Work out the finished part from the listing and answer in its coordinate system (mm). A direction names the side the tool comes from. Coordinates: 2 decimals unless noted, no trailing zeros. Order: outer loops, then holes, each group sorted by start corner. A loop starts at its lowest first (then second) coordinate and runs counter-clockwise, first axis right, second up. Notation, with made-up numbers: M -10.5,22 L 4.5,22 A27 ccw 4.5,38 Z; hole C 70.5,0 d2. An arc over 180 degrees is marked long. Use a Markdown table: item, result.
from build123d import *

# Parameters (mm, degrees)
BOSS_EXTRUDE1_DEPTH     = 6.35
CUT_EXTRUDE1_DEPTH      = 244.131209432
CUT_EXTRUDE1_DEPTH_BACK = 244.131209432
SKETCH4_W               = 101.6
SKETCH4_H               = 101.6
SKETCH4_W_2             = 22.606
SKETCH4_H_2             = 3.302
SKETCH5_W               = 6.888524177
SKETCH5_H               = 88.9
CUT_EXTRUDE2_DEPTH      = 6.35
SKETCH6_R               = 1.429315601
CUT_EXTRUDE3_DEPTH      = 13.97


with BuildPart() as part:
    # Sketch3 → Boss-Extrude1 (new body)
    with BuildSketch(Plane.XY):
        Polygon((0, 77.53985), (0, 55.81015), (5.9944, 55.81015), (5.9944, 34.08045), (0, 34.08045), (0, 12.35075), (0, 0), (25.54605, 0), (25.54605, 5.9944), (47.27575, 5.9944), (47.27575, 0), (69.00545, 0), (69.00545, 5.9944), (90.73515, 5.9944), (90.73515, 0), (112.46485, 0), (112.46485, 5.9944), (134.19455, 5.9944), (134.19455, 0), (155.92425, 0), (155.92425, 5.9944), (177.65395, 5.9944), (177.65395, 0), (203.2, 0), (203.2, 34.08045), (197.2056, 34.08045), (197.2056, 55.81015), (203.2, 55.81015), (203.2, 77.53985), (197.2056, 77.53985), (197.2056, 99.26955), (203.2, 99.26955), (203.2, 120.99925), (203.2, 133.35), (177.65395, 133.35), (177.65395, 127.3556), (155.92425, 127.3556), (155.92425, 133.35), (134.19455, 133.35), (134.19455, 127.3556), (112.46485, 127.3556), (112.46485, 133.35), (90.73515, 133.35), (90.73515, 127.3556), (69.00545, 127.3556), (69.00545, 133.35), (47.27575, 133.35), (47.27575, 127.3556), (25.54605, 127.3556), (25.54605, 133.35), (0, 133.35), (0, 99.26955), (5.9944, 99.26955), (5.9944, 77.53985), align=None)
    extrude(amount=BOSS_EXTRUDE1_DEPTH)

    # Sketch4 → Cut-Extrude1 (cut, two sides: drawn at the far end of the back side and taken through both)
    with BuildSketch(Plane.XY.offset(6.35).offset(-CUT_EXTRUDE1_DEPTH_BACK)):
        with Locations((69.942028986, 69.85)):
            Rectangle(SKETCH4_W, SKETCH4_H)
        with BuildLine():
            ThreePointArc((189.068028986, 120.65), (186.020028986, 123.698), (182.972028986, 120.65))
            Line((182.972028986, 120.65), (189.068028986, 120.65))
        make_face()
        with BuildLine():
            Line((189.068028986, 120.65), (182.972028986, 120.65))
            ThreePointArc((182.972028986, 120.65), (186.020028986, 117.602), (189.068028986, 120.65))
        make_face()
        with BuildLine():
            ThreePointArc((176.368028986, 120.65), (173.320028986, 123.698), (170.272028986, 120.65))
            Line((170.272028986, 120.65), (176.368028986, 120.65))
        make_face()
        with BuildLine():
            Line((176.368028986, 120.65), (170.272028986, 120.65))
            ThreePointArc((170.272028986, 120.65), (173.320028986, 117.602), (176.368028986, 120.65))
        make_face()
        with Locations((164.557028986, 20.701)):
            Rectangle(SKETCH4_W_2, SKETCH4_H_2)
    extrude(amount=CUT_EXTRUDE1_DEPTH + CUT_EXTRUDE1_DEPTH_BACK, mode=Mode.SUBTRACT)

    # Sketch5 → Cut-Extrude2 (cut)
    with BuildSketch(Plane(origin=(0, 0, 0), x_dir=(-1, 0, 0), z_dir=(0, 0, -1))):
        with Locations((-145.073671488, 66.675)):
            Rectangle(SKETCH5_W, SKETCH5_H)
    extrude(amount=-CUT_EXTRUDE2_DEPTH, mode=Mode.SUBTRACT)

    # Sketch6 → Cut-Extrude3 (cut)
    with BuildSketch(Plane.XY.offset(6.35)):
        with Locations((8.25, 95.142010497)):
            Circle(SKETCH6_R)
        with Locations((8.25, 69.742010497)):
            Circle(SKETCH6_R)
        with Locations((8.25, 44.342010497)):
            Circle(SKETCH6_R)
    extrude(amount=-CUT_EXTRUDE3_DEPTH, mode=Mode.SUBTRACT)


solid = part.part
1. For a pull along Y with two mould halves and no side action, classify faces 6 (the face through (164, 19.05, 3)), 7 (the face through (148.518, 66, 3)), 8 (the face through (102, 133.35, 3)), 9 (the face through (112.465, 130, 3)) as +Y half, -Y half, draft (parallel to the pull), parting line (faces both ways), or undercut.
Answers below:
| item | result |
|---|---|
| face 6 | undercut |
| face 7 | undercut |
| face 8 | +Y half |
| face 9 | draft |
2. Section C-C on z = 2.5 is taken. Give the number of separate pieces and of enclosed holes in the cut face, then the cut area to 3 significant figures.
Answers below:
| item | result |
|---|---|
| separate pieces | 1 |
| enclosed holes | 8 |
| area | 14,400 mm² |
3. For faces 1 (the face through (47.276, 3, 3)), 2 (the face through (200, 77.54, 3)), 3 (the face through (120.742, 69, 3)), 4 (the face through (3, 34.08, 3)), 5 (the face through (134.195, 130, 3)), determine the directions among +Z, -Z, +X, -X, +Y, -Y from which every point of the face is accessible in a straight line to the end or side of a thin tool.
Answers below:
| item | result |
|---|---|
| face 1 | +Z, -Z, -Y |
| face 2 | +Z, -Z, +X |
| face 3 | +Z, -Z |
| face 4 | +Z, -Z, -X |
| face 5 | +Z, -Z, +Y |
4. Find the intervals of material crossed by probe 1 along X at (y, z) = (61, 1.75); probe 2 along X at (y, z) = (47, 2); probe 3 along Y at (x, z) = (8.25, 2), in increasing order.
Answers below:
| item | result |
|---|---|
| probe 1 | 0 to 19.14, 120.74 to 141.63, 148.52 to 203.2 |
| probe 2 | 5.99 to 19.14, 120.74 to 141.63, 148.52 to 197.21 |
| probe 3 | 0 to 42.91, 45.77 to 68.31, 71.17 to 93.71, 96.57 to 133.35 |
5. Flat-ended cylindrical pins translate along their axes: P1, Ø5.5, axis at x = 186.02, y = 120.65, coming from the -Z side; P2, Ø1.9, axis at x = 45, z = 1.5, coming from the -Y side; P3, Ø3, axis at y = 53.5, z = 2.5, coming from the -X side. Find the tip coordinate at first contact, or state that the pin passes through.
Answers below:
| item | result |
|---|---|
| P1 | through |
| P2 | y = 5.99 |
| P3 | x = 5.99 |
6. Section B-B on x = 72.5 is taken. Determine the outline of the cut face in (y, z).
Answers below:
| item | result |
|---|---|
| outline | M 5.99,0 L 19.05,0 L 19.05,6.35 L 5.99,6.35 Z; M 120.65,0 L 127.36,0 L 127.36,6.35 L 120.65,6.35 Z |
7. Section A-A on x = 104 is taken. Determine the outline of the cut face in (y, z), then the cut area to 3 significant figures.
Answers below:
| item | result |
|---|---|
| outline | M 0,0 L 19.05,0 L 19.05,6.35 L 0,6.35 Z; M 120.65,0 L 133.35,0 L 133.35,6.35 L 120.65,6.35 Z |
| area | 202 mm² |
